```python
from build123d import *

# Parameters (mm, degrees)
SKETCH1_W           = 609.6
SKETCH1_H           = 76.2
BOSS_EXTRUDE1_DEPTH = 3.175
CUT_EXTRUDE1_DEPTH  = 308.237648246


with BuildPart() as part:
    # Sketch1 → Boss-Extrude1 (new, symmetric)
    with BuildSketch(Plane(origin=(0, 0, 0), x_dir=(1, 0, 0), z_dir=(0, 1, 0))):
        Rectangle(SKETCH1_W, SKETCH1_H)
    extrude(amount=BOSS_EXTRUDE1_DEPTH, both=True)

    # Sketch2 → Cut-Extrude1 (cut, through all)
    with BuildSketch(Plane(origin=(0, 3.175, 0), x_dir=(1, 0, 0), z_dir=(0, 1, 0))):
        with BuildLine():
            Line((-279.4, -4.841875), (279.4, -4.841875))
            ThreePointArc((279.4, -4.841875), (282.178125, -7.62), (279.4, -10.398125))
            Line((279.4, -10.398125), (-279.4, -10.398125))
            ThreePointArc((-279.4, -10.398125), (-282.178125, -7.62), (-279.4, -4.841875))
        make_face()
        with BuildLine():
            Line((-279.4, -23.891875), (279.4, -23.891875))
            ThreePointArc((279.4, -23.891875), (282.178125, -26.67), (279.4, -29.448125))
            Line((279.4, -29.448125), (-279.4, -29.448125))
            ThreePointArc((-279.4, -29.448125), (-282.178125, -26.67), (-279.4, -23.891875))
        make_face()
    extrude(amount=-CUT_EXTRUDE1_DEPTH, mode=Mode.SUBTRACT)


solid = part.part
```
Work out the finished part from the listing and answer in its coordinate system (mm). Give positions to 0.01 mm unless a question says otherwise; leave off trailing zeros. Order: outer loops, then holes, each group sorted by start corner. A loop starts at its lowest first (then second) coordinate and runs counter-clockwise, first axis right, second up. Notation, with made-up numbers: M 37,-17.5 L 53,-17.5 A28 ccw 53,19.5 Z; hole C 65,27.25 d8. An arc over 180 degrees is marked long. Return JSON: item names as keys, results as strings.
1) Section B-B, the plane x = -30.5 is taken. Write down the section's boundary in (y, z) (3 decimals).
Resolved:
{"outline": "M -3.175,-38.1 L 3.175,-38.1 L 3.175,4.842 L -3.175,4.842 Z; M -3.175,10.398 L 3.175,10.398 L 3.175,23.892 L -3.175,23.892 Z; M -3.175,29.448 L 3.175,29.448 L 3.175,38.1 L -3.175,38.1 Z"}
2) Straight lines are drawn through the part: line 1 along Z through (x, y) = (252, -1.25); line 2 along X through (y, z) = (-1.5, 8.5); line 3 along X through (y, z) = (2.5, 27.5). For each, find the intervals that lie inside material, in ascending order. Write a range as [from, to].
Resolved:
{"line 1": "[-38.1, 4.84], [10.4, 23.89], [29.45, 38.1]", "line 2": "[-304.8, -282.04], [282.04, 304.8]", "line 3": "[-304.8, -282.05], [282.05, 304.8]"}
3) Section A-A, the plane y = 1.25 is taken. Write down the section's boundary in (x, z), plus the area to 3 significant figures.
Resolved:
{"outline": "M -304.8,-38.1 L 304.8,-38.1 L 304.8,38.1 L -304.8,38.1 Z; hole M -279.4,4.84 L 279.4,4.84 A2.78 ccw 279.4,10.4 L -279.4,10.4 A2.78 ccw Z; hole M -279.4,23.89 L 279.4,23.89 A2.78 ccw 279.4,29.45 L -279.4,29.45 A2.78 ccw Z", "area": "40,200 mm^2"}
